Verification items for this drawing (mm, ordinates from the low corner). A direction names the side the tool comes from. Give positions to 0.01 mm unless a question says otherwise; leave off trailing zeros. Order: outer loops, then holes, each group sorted by start corner. A loop starts at its lowest first (then second) coordinate and runs counter-clockwise, first axis right, second up.
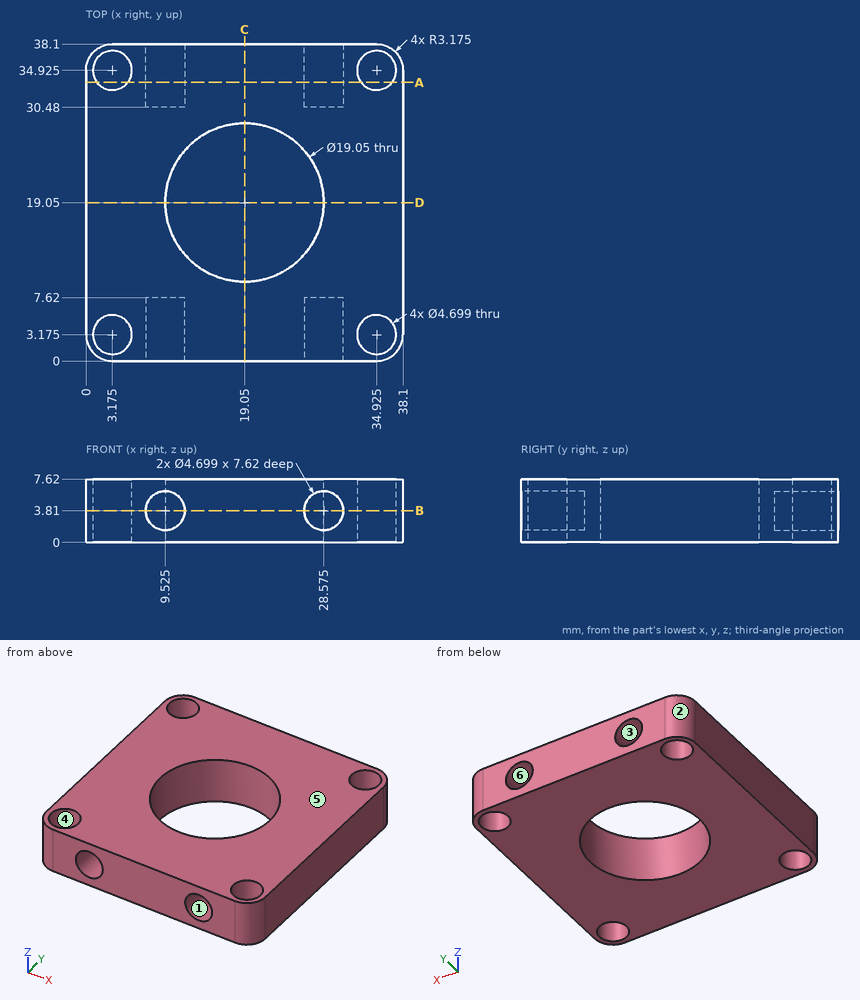
Q1. Cross-section at B-B, the plane z = 3.81. Give the number of separate pieces and of enclosed holes in the cut face, and give its area (3 significant figures).
Q2. Gauge pin test, flat ends, axial feed: P1, Ø1, axis at x = 6.5, z = 4.5, coming from the -Y side; P2, Ø1.4, axis at x = 28.5, z = 4.5, coming from the +Y side; P3, Ø1.4, axis at x = 28.5, z = 4.5, coming from the -Y side. Record the tip position at first contact, or that the pin passes through.
Q3. Access from +Z, -Z, +X, -X, +Y, -Y to the whole of each face (thin tool, end or side, straight path). Record for the marked faces 1 and 2.
Q4. Release check for a two-part mould opening along Z. For the marked faces 3, 4, 5 and 6 record: pulls with the +Z half, pulls with the -Z half, needs draft (parallel to the pull), parting line crosses it, or undercut.
Q5. Cross-section at A-A, the plane y = 33.5. Record the boundary of the cut face in (x, z) (1 decimal), and give its area (3 significant figures).
Q6. Cross-section at C-C, the plane x = 19.05. Record the boundary of the cut face in (y, z) (3 decimals).
Q7. Thickness scan on L1, parallel to Y at x = 35, z = 3; L2, parallel to X at y = 36.5, z = 3.81; L3, parallel to Y at x = 19, z = 7.25. Record the ranges inside material, lowest first.
Answers follow:
1. separate pieces: 1
1. enclosed holes: 5
1. area: 945 mm2
2. P1: stops at y = 0
2. P2: stops at y = 30.48
2. P3: stops at y = 7.62
3. face 1: -Y
3. face 2: +Z, -Z, -X, +Y
4. face 3: undercut
4. face 4: needs draft
4. face 5: pulls with the +Z half
4. face 6: undercut
5. outline: (0, 0) - (1.3, 0) - (1.3, 7.6) - (0, 7.6) - close; (5, 0) - (33.1, 0) - (33.1, 7.6) - (5, 7.6) - close; (36.8, 0) - (38.1, 0) - (38.1, 7.6) - (36.8, 7.6) - close; hole circle Ø4.7 at (9.5, 3.8); hole circle Ø4.7 at (28.6, 3.8)
5. area: 199 mm2
6. outline: (0, 0) - (9.525, 0) - (9.525, 7.62) - (0, 7.62) - close; (28.575, 0) - (38.1, 0) - (38.1, 7.62) - (28.575, 7.62) - close
7. L1: y = 0 to 0.83, 5.52 to 32.58, 37.27 to 38.1
7. L2: x = 0.42 to 1.43, 4.92 to 7.18, 11.87 to 26.23, 30.92 to 33.18, 36.67 to 37.68
7. L3: y = 0 to 9.53, 28.57 to 38.1
